Geometry check sheet. Reference: the model listing, model coordinates, mm. Face numbers are marked on the shaded views. A direction names the side the tool comes from. Coordinates: 2 decimals unless noted, no trailing zeros. Loops run counter-clockwise (first coordinate to the right, second up) from the corner with the lowest first, then second, coordinate; pieces in that order, holes last.
from build123d import *

# Parameters (mm, degrees)
F1_DEPTH = 510
F3_DEPTH = 2370


with BuildPart() as f1:
    # F0 (on Front) → F1 (new body)
    with BuildSketch(Plane.XZ):
        Polygon((450, 800), (0, 800), (-450, 800), (-450, 0), (-350, 0), (-350, 700), (0, 700), (350, 700), (350, 0), (450, 0), align=None)
    extrude(amount=F1_DEPTH)

    # F2 (on Front) → F3 (join)
    with BuildSketch(Plane.XZ):
        Polygon((-450, 0), (0, 0), (450, 0), (450, 1), (-450, 1), align=None)
    extrude(amount=F3_DEPTH)


solid = f1.part
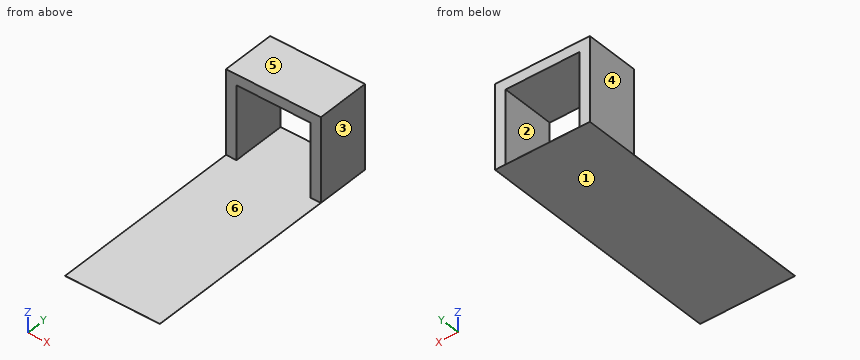
1) Section check C-C on y = -392. Record the cut outline in (x, z).
Data:
outline: (-450, 0) - (450, 0) - (450, 800) - (-450, 800) - close; hole (-350, 1) - (350, 1) - (350, 700) - (-350, 700) - close
2) Section check D-D on x = -384. Record the cut outline in (y, z), and give its area (3 significant figures).
Data:
outline: (-2370, 0) - (0, 0) - (0, 800) - (-510, 800) - (-510, 1) - (-2370, 1) - close
area: 410,000 mm2
3) Section check A-A on x = -88. Record the cut outline in (y, z).
Data:
outline: (-2370, 0) - (0, 0) - (0, 1) - (-2370, 1) - close; (-510, 700) - (0, 700) - (0, 800) - (-510, 800) - close
4) Access from +Z, -Z, +X, -X, +Y, -Y to the whole of each face (thin tool, end or side, straight path). Record for the marked faces 1 and 2.
Data:
face 1: -Z, +X, -X, +Y, -Y
face 2: +Y, -Y
5) Depth check by flat-ended pin: pin 1 (12 mm diameter, centred on x = -317, y = -950, fed in from -Z); pin 2 (10 mm diameter, centred on x = 90, y = -1219.5, fed in from +Z). Enter the tip coordinate at first touch or a pass-through.
Data:
pin 1: stops at z = 0
pin 2: stops at z = 1
6) Material ranges on probe 1 along X at (y, z) = (-210.5, 259); probe 2 along Z at (x, y) = (-124, -102); probe 3 along Z at (x, y) = (404, -2225), recorded low to high.
Data:
probe 1: x = -450 to -350, 350 to 450
probe 2: z = 0 to 1, 700 to 800
probe 3: z = 0 to 1
7) Mould release check, pull along X, two halves, no side actions. Record for the marked faces 3, 4, 5 and 6: +X half, -X half, draft (parallel to the pull), parting line (faces both ways), or undercut.
Data:
face 3: +X half
face 4: -X half
face 5: draft
face 6: undercut
8) Section check B-B on z = 398.5. Record the cut outline in (x, y).
Data:
outline: (-450, -510) - (-350, -510) - (-350, 0) - (-450, 0) - close; (350, -510) - (450, -510) - (450, 0) - (350, 0) - close
